The listing builds one solid part. Answer for the finished solid, in the listing's coordinates (mm). Coordinates: 2 decimals unless noted, no trailing zeros. Loops run counter-clockwise (first coordinate to the right, second up) from the corner with the lowest first, then second, coordinate; pieces in that order, holes last. Notation, with made-up numbers: (44, 41.5) - (90, 41.5) arc R14 cw to (90, 48.5) - close; hole circle Ø10 at (-31, 64.25). An arc over 180 degrees is marked (long way). One line per question, with ' | ' between items.
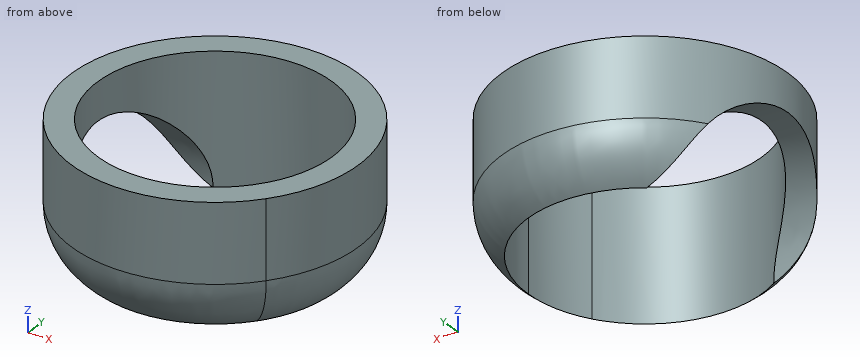
from build123d import *

# Parameters (mm, degrees)
F1_DEPTH    = 10
F3_DEPTH    = 25
F4_DEPTH    = 25
F5_T2_ANGLE = 228.5604314435
F5_T4_ANGLE = 149.7338838055


# Not quite as in the source:
# - a fillet or chamfer that OpenCascade refuses, or shapes differently, is made with other operations: its cross-section is extruded or revolved along the edge and cut away or added


with BuildPart() as f1:
    # F0 (on Top) → F1 (new body)
    with BuildSketch(Plane.XY):
        with BuildLine():
            ThreePointArc((7.4897676428, -4.9903287123), (-9, 0), (7.4897676428, 4.9903287123))
            ThreePointArc((7.4897676428, 4.9903287123), (8.0061615463, 5.944514107), (8.6101788512, 6.8457884973))
            ThreePointArc((8.6101788512, 6.8457884973), (-11, 0), (8.6101788512, -6.8457884973))
            ThreePointArc((8.6101788512, -6.8457884973), (8.0061615463, -5.944514107), (7.4897676428, -4.9903287123))
        make_face()
        with BuildLine():
            ThreePointArc((7.4897676428, 4.9903287123), (8.6141717183, 2.6069226316), (9, 0))
            ThreePointArc((9, 0), (8.6141717183, -2.6069226316), (7.4897676428, -4.9903287123))
            ThreePointArc((7.4897676428, -4.9903287123), (8.0061615463, -5.944514107), (8.6101788512, -6.8457884973))
            ThreePointArc((8.6101788512, -6.8457884973), (11, 0), (8.6101788512, 6.8457884973))
            ThreePointArc((8.6101788512, 6.8457884973), (8.0061615463, 5.944514107), (7.4897676428, 4.9903287123))
        make_face()
    extrude(amount=F1_DEPTH)

    # F2 (on Right) → F3 (cut)
    with BuildSketch(Plane.YZ):
        with BuildLine():
            add(Edge.make_bspline(
                [(-7.6260738851, 0), (-7.6289822236, 4.6128164915), (0.0415342584, 9.6458716707), (7.41270182, 4.5238972991), (7.3739261149, 0)],
                knots=[0, 0, 0, 0, 0.502214143, 1, 1, 1, 1], degree=3))
            Line((-7.6260738851, 0), (7.3739261149, 0))
        make_face()
    extrude(amount=-F3_DEPTH, mode=Mode.SUBTRACT)

    # F2 (on Right) → F4 (cut)
    with BuildSketch(Plane.YZ):
        with BuildLine():
            add(Edge.make_bspline(
                [(-7.6260738851, 0), (-7.6289822236, 4.6128164915), (0.0415342584, 9.6458716707), (7.41270182, 4.5238972991), (7.3739261149, 0)],
                knots=[0, 0, 0, 0, 0.502214143, 1, 1, 1, 1], degree=3))
            Line((-7.6260738851, 0), (7.3739261149, 0))
        make_face()
    extrude(amount=-F4_DEPTH, mode=Mode.SUBTRACT)

    # F5: fillet of radius 5 on 2 edges, made by hand

    # F5_s1 → F5_t2 (revolve, cut)
    with BuildSketch(Plane(origin=(0, 0, 0), x_dir=(0, 0, 1), z_dir=(-0.6223444088, -0.7827435319, 0))):
        with BuildLine():
            ThreePointArc((0, -9), (1.7639320225, -10.472135955), (4, -11))
            Line((4, -11), (0, -11))
            Line((0, -11), (0, -9))
        make_face()
    revolve(axis=Axis((0, 0, 0), (0, 0, 1)), revolution_arc=F5_T2_ANGLE, mode=Mode.SUBTRACT)

    # F5_s3 → F5_t4 (revolve, cut)
    with BuildSketch(Plane(origin=(0, 0, 0), x_dir=(0, 0, 1), z_dir=(0.1429989905, 0.9897228343, 0))):
        with BuildLine():
            ThreePointArc((0, -9), (1.7639320225, -10.472135955), (4, -11))
            Line((4, -11), (0, -11))
            Line((0, -11), (0, -9))
        make_face()
    revolve(axis=Axis((0, 0, 0), (0, 0, 1)), revolution_arc=F5_T4_ANGLE, mode=Mode.SUBTRACT)


solid = f1.part
Item 1: Each of these flat-tipped pins is pushed along its axis until it touches: pin 1 Ø2 at (y, z) = (-4, 3.5) entering from -X; pin 2 Ø3 at (x, z) = (1.5, 4) entering from +Y; pin 3 Ø3 at (y, z) = (-6.5, 5) entering from -X; pin 4 Ø1.5 at (x, z) = (2.5, 2) entering from -Y. Where does it stop, or does it pass through?
Taken from the geometry:
pin 1: stops at x = 7.48 | pin 2: stops at y = 11 | pin 3: stops at x = -9.77 | pin 4: stops at y = -10.6
Item 2: Find section A-A, the plane x = 0. Write down the section's boundary in (y, z).
Taken from the geometry:
outline: (-11, 4) arc R5 ccw to (-9, 0) - (-9, 10) - (-11, 10) - close; (9, 0) arc R5 ccw to (11, 4) - (11, 10) - (9, 10) - close
Item 3: Find the intervals of material crossed by line 1 (Y direction, x = 0, z = 6.5); line 2 (X direction, y = 0, z = 4.5); line 3 (Y direction, x = -2.75, z = 4.75), in increasing order. Write a range as [from, to].
Taken from the geometry:
line 1: y = [-11, -9], [9, 11] | line 2: x = [9, 11] | line 3: y = [-10.65, -8.57], [8.57, 10.65]
Item 4: Find section B-B, the plane z = 9. Write down the section's boundary in (x, y), plus the area to 3 significant figures.
Taken from the geometry:
outline: circle Ø22 at (0, 0); hole circle Ø18 at (0, 0) | area: 126 mm2
